```python
from build123d import *

# Parameters (mm, degrees)
F0_R     = 2.6035
F1_DEPTH = 6.35


with BuildPart() as f1:
    # F0 (on Right) → F1 (new body)
    with BuildSketch(Plane.YZ):
        with BuildLine():
            Line((-24.071991, 17.426708), (-24.071991, -17.426708))
            Line((-24.071991, -17.426708), (-24.071991, -18.031692))
            ThreePointArc((-24.071991, -18.031692), (-22.111076, -22.325031), (-17.7292, -24.0792))
            Line((-17.7292, -24.0792), (17.7292, -24.0792))
            Line((17.7292, -24.0792), (79.226878, -24.0792))
            ThreePointArc((79.226878, -24.0792), (83.717007, -22.219328), (85.576878, -17.7292))
            Line((85.576878, -17.7292), (85.576878, 17.7292))
            ThreePointArc((85.576878, 17.7292), (83.717007, 22.219328), (79.226878, 24.0792))
            Line((79.226878, 24.0792), (17.7292, 24.0792))
            Line((17.7292, 24.0792), (-17.7292, 24.0792))
            ThreePointArc((-17.7292, 24.0792), (-22.111076, 22.325031), (-24.071991, 18.031692))
            Line((-24.071991, 18.031692), (-24.071991, 17.426708))
        make_face()
        with Locations((-17.7292, -17.7292)):
            Circle(F0_R, mode=Mode.SUBTRACT)
        with BuildLine():
            ThreePointArc((0, -10.363654), (1.259078, -10.623975), (2.311689, -11.362253))
            Line((2.311689, -11.362253), (8.776098, -18.2285))
            ThreePointArc((8.776098, -18.2285), (9.077593, -19.946239), (7.620254, -20.9042))
            Line((7.620254, -20.9042), (0, -20.9042))
            Line((0, -20.9042), (-7.620254, -20.9042))
            ThreePointArc((-7.620254, -20.9042), (-9.077593, -19.946239), (-8.776098, -18.2285))
            Line((-8.776098, -18.2285), (-2.311689, -11.362253))
            ThreePointArc((-2.311689, -11.362253), (-1.259078, -10.623975), (0, -10.363654))
        make_face(mode=Mode.SUBTRACT)
        with BuildLine():
            ThreePointArc((20.3327, -17.7292), (15.888247, -19.570153), (17.7292, -15.1257))
            ThreePointArc((17.7292, -15.1257), (19.570153, -15.888247), (20.3327, -17.7292))
        make_face(mode=Mode.SUBTRACT)
        with BuildLine():
            Line((51.978643, -20.9042), (27.838146, -20.9042))
            ThreePointArc((27.838146, -20.9042), (26.380807, -19.946239), (26.682302, -18.2285))
            Line((26.682302, -18.2285), (40.366631, -3.693533))
            ThreePointArc((40.366631, -3.693533), (41.946698, -3.251965), (43.073684, -4.444231))
            ThreePointArc((43.073684, -4.444231), (46.530538, -12.207495), (52.791839, -17.953297))
            ThreePointArc((52.791839, -17.953297), (53.509094, -19.738454), (51.978643, -20.9042))
        make_face(mode=Mode.SUBTRACT)
        with BuildLine():
            ThreePointArc((75.021357, -20.9042), (73.490906, -19.738454), (74.208161, -17.953297))
            ThreePointArc((74.208161, -17.953297), (77.097094, -15.877802), (79.592302, -13.342541))
            ThreePointArc((79.592302, -13.342541), (81.352946, -12.862443), (82.401878, -14.355796))
            Line((82.401878, -14.355796), (82.401878, -19.3167))
            ThreePointArc((82.401878, -19.3167), (81.93691, -20.439232), (80.814378, -20.9042))
            Line((80.814378, -20.9042), (75.021357, -20.9042))
        make_face(mode=Mode.SUBTRACT)
        with BuildLine():
            Line((-10.998523, 2.734687), (-10.998523, -2.734687))
            ThreePointArc((-10.998523, -2.734687), (-11.830222, -5.87648), (-14.107455, -8.195271))
            Line((-14.107455, -8.195271), (-18.572501, -10.845448))
            ThreePointArc((-18.572501, -10.845448), (-20.168216, -10.859878), (-20.970268, -9.480302))
            Line((-20.970268, -9.480302), (-20.970268, 9.480302))
            ThreePointArc((-20.970268, 9.480302), (-20.168216, 10.859878), (-18.572501, 10.845448))
            Line((-18.572501, 10.845448), (-14.107455, 8.195271))
            ThreePointArc((-14.107455, 8.195271), (-11.830222, 5.87648), (-10.998523, 2.734687))
        make_face(mode=Mode.SUBTRACT)
        with Locations((-17.7292, 17.7292)):
            Circle(F0_R, mode=Mode.SUBTRACT)
        Polygon((-5.499261, 3.175), (0, 6.35), (5.499261, 3.175), (5.499261, -3.175), (0, -6.35), (-5.499261, -3.175), align=None, mode=Mode.SUBTRACT)
        with BuildLine():
            Line((14.107455, 8.195271), (17.7292, 10.344917))
            Line((17.7292, 10.344917), (18.197877, 10.623095))
            ThreePointArc((18.197877, 10.623095), (18.588032, 10.788851), (19.008143, 10.845448))
            Line((19.008143, 10.845448), (22.932392, 10.845448))
            ThreePointArc((22.932392, 10.845448), (23.352503, 10.788851), (23.742659, 10.623095))
            Line((23.742659, 10.623095), (27.83308, 8.195271))
            ThreePointArc((27.83308, 8.195271), (30.110313, 5.87648), (30.942013, 2.734687))
            Line((30.942013, 2.734687), (30.942013, -2.734687))
            ThreePointArc((30.942013, -2.734687), (30.110313, -5.87648), (27.83308, -8.195271))
            Line((27.83308, -8.195271), (23.742659, -10.623095))
            ThreePointArc((23.742659, -10.623095), (23.352503, -10.788851), (22.932392, -10.845448))
            Line((22.932392, -10.845448), (19.008143, -10.845448))
            ThreePointArc((19.008143, -10.845448), (18.588032, -10.788851), (18.197877, -10.623095))
            Line((18.197877, -10.623095), (17.7292, -10.344917))
            Line((17.7292, -10.344917), (14.107455, -8.195271))
            ThreePointArc((14.107455, -8.195271), (11.830222, -5.87648), (10.998523, -2.734687))
            Line((10.998523, -2.734687), (10.998523, 2.734687))
            ThreePointArc((10.998523, 2.734687), (11.830222, 5.87648), (14.107455, 8.195271))
        make_face(mode=Mode.SUBTRACT)
        with BuildLine():
            ThreePointArc((0, 10.363654), (-1.259078, 10.623975), (-2.311689, 11.362253))
            Line((-2.311689, 11.362253), (-8.776098, 18.2285))
            ThreePointArc((-8.776098, 18.2285), (-9.077593, 19.946239), (-7.620254, 20.9042))
            Line((-7.620254, 20.9042), (0, 20.9042))
            Line((0, 20.9042), (7.620254, 20.9042))
            ThreePointArc((7.620254, 20.9042), (9.077593, 19.946239), (8.776098, 18.2285))
            Line((8.776098, 18.2285), (2.311689, 11.362253))
            ThreePointArc((2.311689, 11.362253), (1.259078, 10.623975), (0, 10.363654))
        make_face(mode=Mode.SUBTRACT)
        with BuildLine():
            ThreePointArc((17.7292, 15.1257), (15.888247, 19.570153), (20.3327, 17.7292))
            ThreePointArc((20.3327, 17.7292), (19.570153, 15.888247), (17.7292, 15.1257))
        make_face(mode=Mode.SUBTRACT)
        with BuildLine():
            ThreePointArc((52.791839, 17.953297), (46.530538, 12.207495), (43.073684, 4.444231))
            ThreePointArc((43.073684, 4.444231), (41.946698, 3.251965), (40.366631, 3.693533))
            Line((40.366631, 3.693533), (26.682302, 18.2285))
            ThreePointArc((26.682302, 18.2285), (26.380807, 19.946239), (27.838146, 20.9042))
            Line((27.838146, 20.9042), (51.978643, 20.9042))
            ThreePointArc((51.978643, 20.9042), (53.509094, 19.738454), (52.791839, 17.953297))
        make_face(mode=Mode.SUBTRACT)
        with BuildLine():
            ThreePointArc((63.5, 14.2875), (73.602788, 10.102788), (77.7875, 0))
            ThreePointArc((77.7875, 0), (53.397212, -10.102788), (63.5, 14.2875))
        make_face(mode=Mode.SUBTRACT)
        with BuildLine():
            ThreePointArc((74.208161, 17.953297), (73.490906, 19.738454), (75.021357, 20.9042))
            Line((75.021357, 20.9042), (80.814378, 20.9042))
            ThreePointArc((80.814378, 20.9042), (81.93691, 20.439232), (82.401878, 19.3167))
            Line((82.401878, 19.3167), (82.401878, 14.355796))
            ThreePointArc((82.401878, 14.355796), (81.352946, 12.862443), (79.592302, 13.342541))
            ThreePointArc((79.592302, 13.342541), (77.097094, 15.877802), (74.208161, 17.953297))
        make_face(mode=Mode.SUBTRACT)
    extrude(amount=F1_DEPTH)


solid = f1.part
```
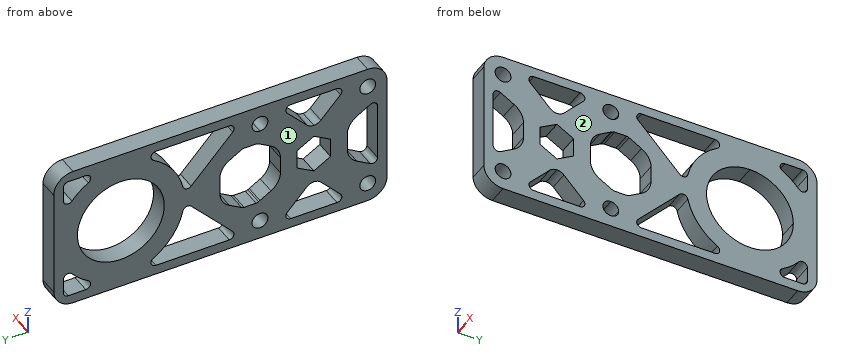
Input: part model. Units: mm. Frame: model coordinates. Face numbers are marked on the shaded views. Give positions to 0.01 mm unless a question says otherwise; leave off trailing zeros. Order: outer loops, then holes, each group sorted by start corner. A loop starts at its lowest first (then second) coordinate and runs counter-clockwise, first axis right, second up. Notation, with made-up numbers: M 80,56.25 L 114,56.25 A18 ccw 114,91.25 Z; hole C 69.25,49 d2. An arc over 180 degrees is marked long. Return JSON: item names as keys, results as strings.
1) Line query: L1, parallel to Y at x = 1, z = 0.5; L2, parallel to Y at x = 1.5, z = -5.5; L3, parallel to Z at x = 4.75, y = 38. Output: solid intervals per line, ascending. Write a range as [from, to].
Taken from the geometry:
{"L1": "y = [-24.07, -20.97], [-11, -5.5], [5.5, 11], [30.94, 49.22], [77.78, 85.58]", "L2": "y = [-24.07, -20.97], [-11.63, -1.47], [1.47, 11.63], [30.31, 38.67], [43.33, 50.31], [76.69, 85.58]", "L3": "z = [-24.08, -20.9], [-6.21, 6.21], [20.9, 24.08]"}
2) Section query C-C on y = 60.5. Output: boundary loops of the cut face in (x, z), and give its area (3 significant figures).
Taken from the geometry:
{"outline": "M 0,-24.08 L 6.35,-24.08 L 6.35,-13.97 L 0,-13.97 Z; M 0,13.97 L 6.35,13.97 L 6.35,24.08 L 0,24.08 Z", "area": "128 mm2"}
3) Section query B-B on z = 1. Output: boundary loops of the cut face in (x, y).
Taken from the geometry:
{"outline": "M 0,-24.07 L 6.35,-24.07 L 6.35,-20.97 L 0,-20.97 Z; M 0,-11 L 6.35,-11 L 6.35,-5.5 L 0,-5.5 Z; M 0,5.5 L 6.35,5.5 L 6.35,11 L 0,11 Z; M 0,30.94 L 6.35,30.94 L 6.35,49.25 L 0,49.25 Z; M 0,77.75 L 6.35,77.75 L 6.35,85.58 L 0,85.58 Z"}
4) Section query A-A on y = 48. Output: boundary loops of the cut face in (x, z).
Taken from the geometry:
{"outline": "M 0,-24.08 L 6.35,-24.08 L 6.35,-20.9 L 0,-20.9 Z; M 0,-14.03 L 6.35,-14.03 L 6.35,14.03 L 0,14.03 Z; M 0,20.9 L 6.35,20.9 L 6.35,24.08 L 0,24.08 Z"}
5) Section query D-D on x = 3.75. Count the separate pieces of the cut face and the enclosed holes in it, and give its area (3 significant figures).
Taken from the geometry:
{"separate pieces": "1", "enclosed holes": "14", "area": "3,010 mm2"}
6) Mould query, pull axis X, two halves, no side actions, for the marked faces 1 and 2. Classes: released by +X, released by -X, zero draft, split by the parting line, or undercut.
Taken from the geometry:
{"face 1": "released by -X", "face 2": "released by +X"}
